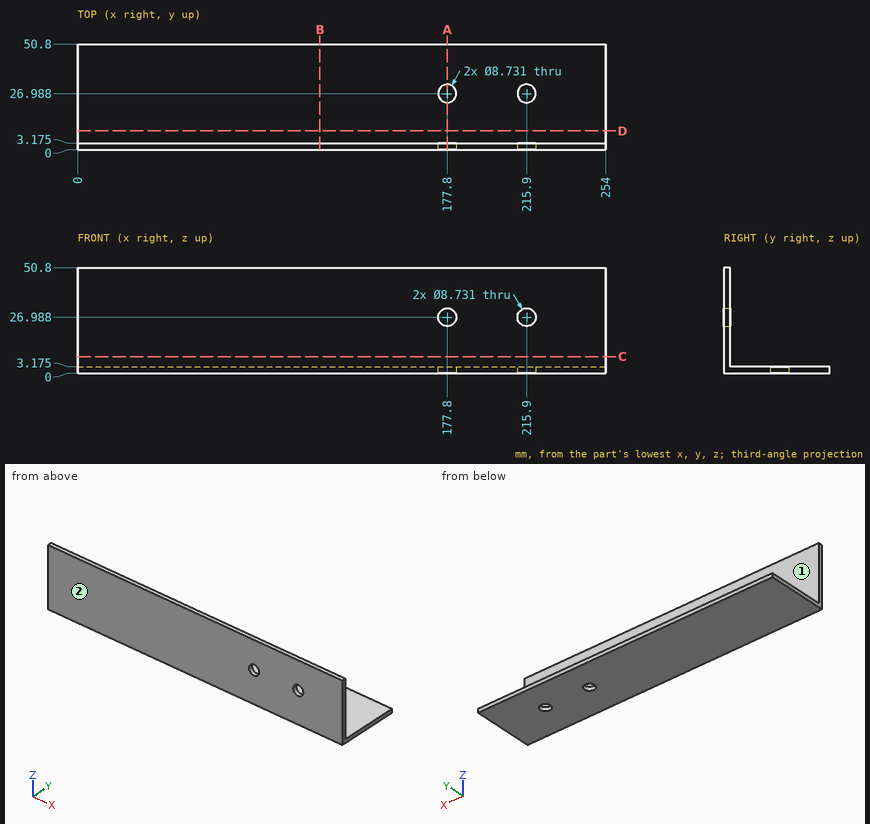
Input: dimensioned drawing with shaded views. Units: mm. Origin: part minimum x, y, z. A direction names the side the tool comes from. Give positions to 0.01 mm unless a question says otherwise; leave off trailing zeros. Loops run counter-clockwise (first coordinate to the right, second up) from the corner with the lowest first, then second, coordinate; pieces in that order, holes last. Notation, with made-up numbers: (0, -32) -> (26, -32) arc R24 cw to (26, 2) -> close; hole circle Ø6 at (20, 13). An arc over 180 degrees is marked (long way). Use a Markdown table: item, result. Add a question column.
1) Section query A-A, the plane x = 177.8. Return the cut outline in (y, z) (1 decimal).
2) Section query C-C, the plane z = 8. Return the cut outline in (x, y) (1 decimal).
3) Reachability of the marked faces 1 and 2 from +Z, -Z, +X, -X, +Y, -Y: full face, straight path, thin tool, end or side. Return the list, or none.
4) Section query B-B, the plane x = 116.5. Return the cut outline in (y, z) (1 decimal).
5) Line query: line 1 along Z through (x, y) = (177.8, 0.85); line 2 along Z through (x, y) = (139.5, 7) (1 decimal). Output: solid intervals per line, ascending. Write a range as [from, to].
6) First-contact query: pin 1 (10 mm diameter, centred on x = 215.9, y = 26.99, fed in from -Z); pin 2 (5 mm diameter, centred on x = 177.8, y = 26.99, fed in from -Z); pin 3 (4 mm diameter, centred on x = 87.5, z = 13.5, fed in from +Y) (1 decimal); pin 4 (24 mm diameter, centred on x = 82.5, y = 18.5, fed in from +Z) (1 decimal). Flat tips, straight axial feed; report the tip coordinate or a pass-through.
Numbers:
| question | item | result |
|---|---|---|
| 1 | outline | (0, 0) -> (22.6, 0) -> (22.6, 3.2) -> (3.2, 3.2) -> (3.2, 22.6) -> (0, 22.6) -> close; (0, 31.4) -> (3.2, 31.4) -> (3.2, 50.8) -> (0, 50.8) -> close; (31.4, 0) -> (50.8, 0) -> (50.8, 3.2) -> (31.4, 3.2) -> close |
| 2 | outline | (0, 0) -> (254, 0) -> (254, 3.2) -> (0, 3.2) -> close |
| 3 | face 1 | +Z, +X, -X, +Y |
| 3 | face 2 | +Z, -Z, +X, -X, -Y |
| 4 | outline | (0, 0) -> (50.8, 0) -> (50.8, 3.2) -> (3.2, 3.2) -> (3.2, 50.8) -> (0, 50.8) -> close |
| 5 | line 1 | z = [0, 22.62], [31.35, 50.8] |
| 5 | line 2 | z = [0, 3.2] |
| 6 | pin 1 | stops at z = 0 |
| 6 | pin 2 | passes through |
| 6 | pin 3 | stops at y = 3.2 |
| 6 | pin 4 | stops at z = 3.2 |
